Build history of the part. All positions in model axes, mm. Face numbers are marked on the shaded views. A direction names the side the tool comes from. Give positions to 0.01 mm unless a question says otherwise; leave off trailing zeros. Write each loop counter-clockwise with the first axis right and the second up, starting at its lowest first coordinate (ties: lowest second). Pieces come first, ordered by that corner, then holes. Notation, with made-up numbers: M 31,36.25 L 44,36.25 A14 cw 44,56.25 Z; hole C 24,-8.75 d3. An arc over 180 degrees is marked long. One line per item, written item: value. Start each with the question number.
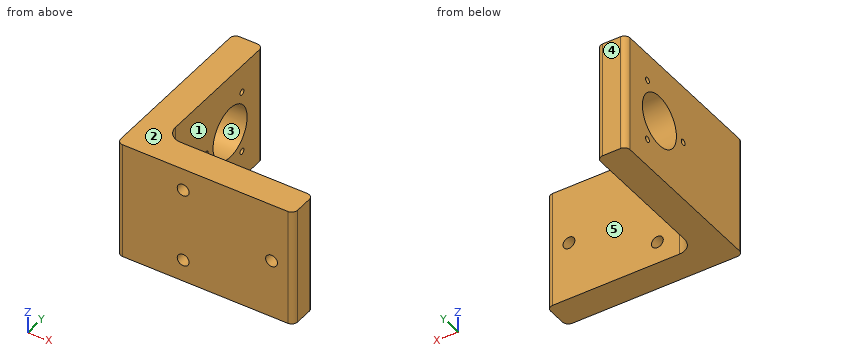
from build123d import *

# Parameters (mm, degrees)
BOSS_EXTRUDE1_DEPTH     = 50.8
FILLET1_R               = 2.54
FILLET2_R               = 6.35
SKETCH2_R               = 11.1125
CUT_EXTRUDE1_DEPTH      = 112.44204772
M3X0_5_TAPPED_HOLE1_D   = 2.5
F_1_4_20_TAPPED_HOLE1_D = 5.1054


with BuildPart() as part:
    # Sketch1 → Boss-Extrude1 (new body)
    with BuildSketch(Plane.XY):
        Polygon((0, 0), (0, 76.2), (12.7, 76.2), (12.7, 12.7), (76.2, 12.7), (76.2, 0), align=None)
    extrude(amount=BOSS_EXTRUDE1_DEPTH)

    # Fillet1
    fillet1_edges = [part.edges().sort_by_distance(p)[0] for p in [
        (0, 0, 25.4),
        (0, 76.2, 25.4),
        (12.7, 76.2, 25.4),
        (76.2, 12.7, 25.4),
        (76.2, 0, 25.4),
    ]]
    fillet(fillet1_edges, radius=FILLET1_R)

    # Fillet2
    fillet2_edges = [part.edges().sort_by_distance(p)[0] for p in [
        (12.7, 12.7, 25.4),
    ]]
    fillet(fillet2_edges, radius=FILLET2_R)

    # Sketch2 → Cut-Extrude1 (cut, through all)
    with BuildSketch(Plane(origin=(12.7, 0, 0), x_dir=(0, 0, -1), z_dir=(1, 0, 0))):
        with Locations(Location((-25.4, 54.61, 0), (0, 0, 90))):
            Circle(SKETCH2_R)
    extrude(amount=-CUT_EXTRUDE1_DEPTH, mode=Mode.SUBTRACT)

    # M3x0.5 Tapped Hole1 (through all)
    with Locations(Plane(origin=(12.7, 0, 0), x_dir=(0, 0, -1), z_dir=(1, 0, 0))):
        with Locations((-38.823393759, 62.36), (-11.976606241, 62.36), (-25.601459668, 39.111309281)):
            Hole(M3X0_5_TAPPED_HOLE1_D / 2)

    # 1/4-20 Tapped Hole1 (through all)
    with Locations(Plane(origin=(0, 12.7, 0), x_dir=(1, 0, 0), z_dir=(0, 1, 0))):
        with Locations((28.575, -9.525), (28.575, -41.275), (66.675, -25.4)):
            Hole(F_1_4_20_TAPPED_HOLE1_D / 2)


solid = part.part
1) Band-saw the part on C-C (y = 62.36). List the corners of the cut face in (x, z).
2) Tool access for the marked faces 4 and 5: list every direction of +Z, -Z, +X, -X, +Y, -Y with a clear straight run to the whole face (end or side of a thin tool).
3) Band-saw the part on D-D (z = 25.4). List the corners of the cut face in (x, y), then the cut area to 3 significant figures.
4) Drop flat-ended pins along their axis: P1, Ø4, axis at x = 30.5, z = 34.5, coming from the -Y side; P2, Ø15, axis at x = 41.5, z = 14.5, coming from the +Y side. Give the stop position or say it passes through.
5) Band-saw the part on B-B (z = 17). List the corners of the cut face in (x, y), then the cut area to 3 significant figures.
6) Mould opens along Z. For the marked faces 1, 2 and 3 say: released by +Z, released by -Z, zero draft, split by the parting line, or undercut.
7) Probe line 1 along Y through (x, z) = (9.5, 26.5); line 2 along Z through (x, y) = (5.5, 54.61); line 3 along Y through (x, z) = (23, 35). List the from-to ranges inside material, lowest first. Write a range as from..to.
8) Band-saw the part on A-A (y = 54.61). List the corners of the cut face in (x, z).
Model answer:
1. outline: M 0,0 L 12.7,0 L 12.7,10.73 L 0,10.73 Z; M 0,13.23 L 12.7,13.23 L 12.7,17.44 L 0,17.44 Z; M 0,33.36 L 12.7,33.36 L 12.7,37.57 L 0,37.57 Z; M 0,40.07 L 12.7,40.07 L 12.7,50.8 L 0,50.8 Z
2. face 4: +Z, -Z, +X, -X, +Y
2. face 5: +Z, -Z, +X, +Y
3. outline: M 0,2.54 A2.54 ccw 2.54,0 L 64.12,0 L 64.12,12.7 L 19.05,12.7 A6.35 cw 12.7,19.05 L 12.7,37.88 L 0,37.88 Z; M 0,40.34 L 12.7,40.34 L 12.7,43.5 L 0,43.5 Z; M 0,65.72 L 12.7,65.72 L 12.7,73.66 A2.54 ccw 10.16,76.2 L 2.54,76.2 A2.54 ccw 0,73.66 Z; M 69.23,0 L 73.66,0 A2.54 ccw 76.2,2.54 L 76.2,10.16 A2.54 ccw 73.66,12.7 L 69.23,12.7 Z
3. area: 1,400 mm²
4. P1: stops at y = 0
4. P2: stops at y = 12.7
5. outline: M 0,2.54 A2.54 ccw 2.54,0 L 73.66,0 A2.54 ccw 76.2,2.54 L 76.2,10.16 A2.54 ccw 73.66,12.7 L 19.05,12.7 A6.35 cw 12.7,19.05 L 12.7,47.33 L 0,47.33 Z; M 0,61.89 L 12.7,61.89 L 12.7,73.66 A2.54 ccw 10.16,76.2 L 2.54,76.2 A2.54 ccw 0,73.66 Z
5. area: 1,590 mm²
6. face 1: zero draft
6. face 2: released by +Z
6. face 3: undercut
7. line 1: y = 0..38.24, 39.98..43.55, 65.67..76.2
7. line 2: z = 0..14.29, 36.51..50.8
7. line 3: y = 0..12.7
8. outline: M 0,0 L 12.7,0 L 12.7,14.29 L 0,14.29 Z; M 0,36.51 L 12.7,36.51 L 12.7,50.8 L 0,50.8 Z
